Read the model definition and answer for the solid it produces. Units are mm, in the model's axes. Give positions to 0.01 mm unless a question says otherwise; leave off trailing zeros. Write each loop counter-clockwise with the first axis right and the second up, starting at its lowest first coordinate (ties: lowest second). Pieces come first, ordered by that corner, then holes.
```python
from build123d import *

# Parameters (mm, degrees)
SKETCH_1_R      = 3.15
EXTRUDE_1_DEPTH = 8
FILLET_1_R      = 0.1
FILLET_2_R      = 0.1


with BuildPart() as part:
    # Эскиз1 → Бобышка-Вытянуть1 (new body)
    with BuildSketch(Plane(origin=(0, 0, 0), x_dir=(1, 0, 0), z_dir=(0, 1, 0))):
        Circle(SKETCH_1_R)
    extrude(amount=EXTRUDE_1_DEPTH)

    # Скругление1
    fillet_1_edges = [part.edges().sort_by_distance(p)[0] for p in [
        (-3.15, 8, 0),
    ]]
    fillet(fillet_1_edges, radius=FILLET_1_R)

    # Скругление2
    fillet_2_edges = [part.edges().sort_by_distance(p)[0] for p in [
        (-3.15, 0, 0),
    ]]
    fillet(fillet_2_edges, radius=FILLET_2_R)


solid = part.part
```
Item 1: Section A-A (y = 1.75) is taken. Write down the section's boundary in (x, z).
Result set:
outline: circle Ø6.3 at (0, 0)
Item 2: Find the intervals of material crossed by line 1 along X through (y, z) = (3, -2); line 2 along Z through (x, y) = (-2.5, 3.25); line 3 along Z through (x, y) = (1, 7), in increasing order.
Result set:
line 1: x = -2.43 to 2.43
line 2: z = -1.92 to 1.92
line 3: z = -2.99 to 2.99
Item 3: Each of these flat-tipped pins is pushed along its axis until it touches: pin 1 Ø2 at (x, y) = (-2, 1.5) entering from -Z; pin 2 Ø1 at (x, y) = (-2.5, 6.5) entering from -Z. Where does it stop, or does it pass through?
Result set:
pin 1: stops at z = -2.99
pin 2: stops at z = -2.43
